Source: three-view drawing plus pictorial views. Frame: mm from the lowest corner of the part. A direction names the side the tool comes from. Round coordinates to 2 decimals unless told otherwise and drop trailing zeros. Loops run counter-clockwise (first coordinate to the right, second up) from the corner with the lowest first, then second, coordinate; pieces in that order, holes last. Notation, with made-up numbers: M 22,16.25 L 50,16.25 A12 ccw 50,37.25 Z; hole C -39,17 d5. An arc over 180 degrees is marked long. Answer as a JSON object with one key per item and string values.
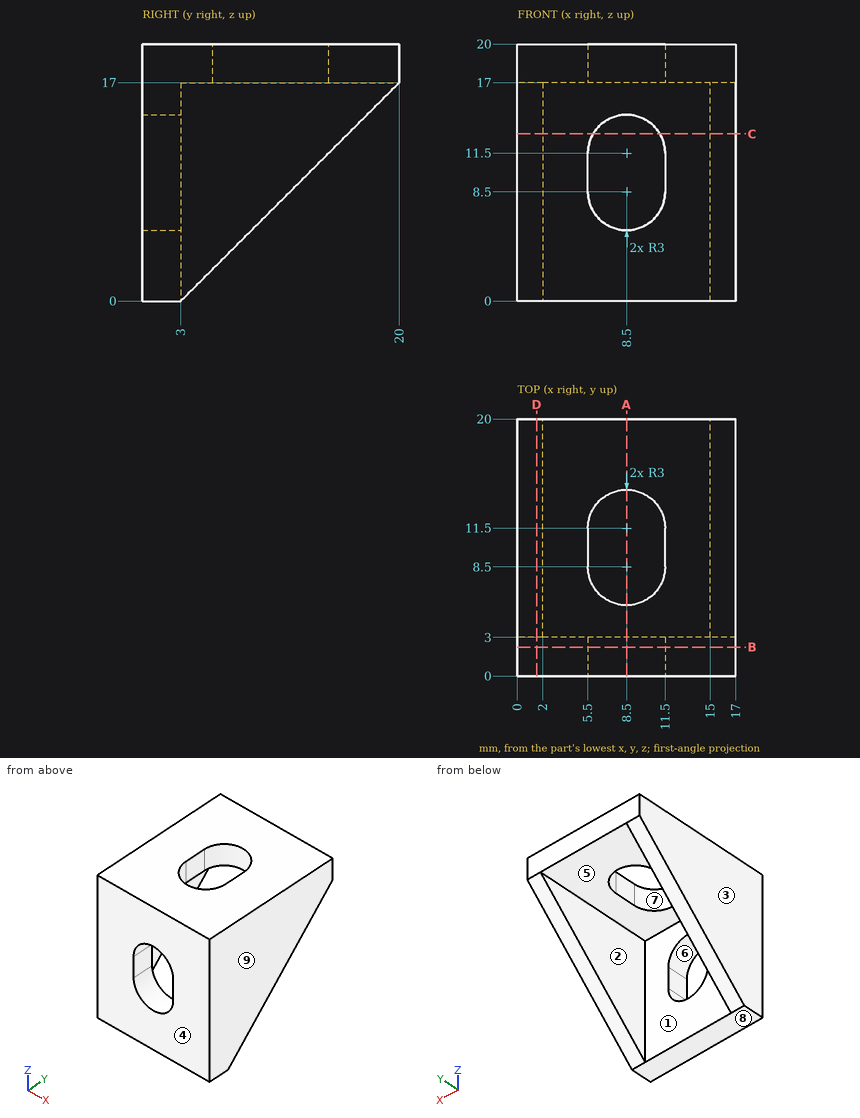
1) Pull-direction query (X, two-part tool) for the marked faces 1, 2, 3 and 4; classes: +X half, -X half, draft (parallel to the pull), parting line (faces both ways), or undercut.
Geometry results:
{"face 1": "undercut", "face 2": "undercut", "face 3": "-X half", "face 4": "draft"}
2) Line query: probe 1 along X at (y, z) = (5.5, 15.75); probe 2 along Z at (x, y) = (1.25, 14.5); probe 3 along Z at (x, y) = (12.5, 11). Output: solid intervals per line, ascending.
Geometry results:
{"probe 1": "0 to 2, 15 to 17", "probe 2": "11.5 to 20", "probe 3": "17 to 20"}
3) Cut plane A-A on x = 8.5. Return the cut outline in (y, z), and give its area (3 significant figures).
Geometry results:
{"outline": "M 0,0 L 3,0 L 3,5.5 L 0,5.5 Z; M 0,14.5 L 3,14.5 L 3,17 L 5.5,17 L 5.5,20 L 0,20 Z; M 14.5,17 L 20,17 L 20,20 L 14.5,20 Z", "area": "57.0 mm2"}
4) Set-up query: the marked faces 5, 6, 7, 8 and 9. Return all of +Z, -Z, +X, -X, +Y, -Y with unobstructed straight access to the full face (end or side cutting, diameter ignored); none if empty.
Geometry results:
{"face 5": "-Z, +Y", "face 6": "+Y, -Y", "face 7": "+Z, -Z", "face 8": "-Z, +X, -X, +Y, -Y", "face 9": "+Z, -Z, +X, +Y, -Y"}
5) First-contact query: pin 1 (6.5 mm diameter, centred on x = 9, z = 6, fed in from +Y); pin 2 (1.5 mm diameter, centred on x = 8, y = 16, fed in from -Z); pin 3 (4 mm diameter, centred on x = 2, z = 5, fed in from +Y). Flat tips, straight axial feed; report the tip coordinate or a pass-through.
Geometry results:
{"pin 1": "y = 3", "pin 2": "z = 17", "pin 3": "y = 10"}
6) Cut plane C-C on z = 13. Return the cut outline in (x, y), and give its area (3 significant figures).
Geometry results:
{"outline": "M 0,0 L 5.9,0 L 5.9,3 L 2,3 L 2,16 L 0,16 Z; M 11.1,0 L 17,0 L 17,16 L 15,16 L 15,3 L 11.1,3 Z", "area": "87.4 mm2"}
7) Cut plane D-D on x = 1.5. Return the cut outline in (y, z), and give its area (4 significant figures).
Geometry results:
{"outline": "M 0,0 L 3,0 L 20,17 L 20,20 L 0,20 Z", "area": "255.5 mm2"}
8) Cut plane B-B on y = 2.25. Return the cut outline in (x, z), and give its area (3 significant figures).
Geometry results:
{"outline": "M 0,0 L 17,0 L 17,20 L 0,20 Z; hole M 5.5,8.5 A3 ccw 11.5,8.5 L 11.5,11.5 A3 ccw 5.5,11.5 Z", "area": "294 mm2"}
